```python
from build123d import *

# Parameters (mm, degrees)
F0_W      = 50
F0_H      = 81
F1_DEPTH  = 2
F0_H_2    = 3.6
F2_DEPTH  = 3.6
F4_R      = 1.75
F5_DEPTH  = 2
F3_R      = 1.75
F6_DEPTH  = 2
F1_FACE_W = 50
F1_FACE_H = 2
F7_DEPTH  = 6


with BuildPart() as f1:
    # F0 (on Front) → F1 (new body)
    with BuildSketch(Plane.XZ):
        with Locations((25, 40.5)):
            Rectangle(F0_W, F0_H)
    extrude(amount=F1_DEPTH)

    # F0 (on Front) → F2 (join)
    with BuildSketch(Plane.XZ):
        with Locations((25, 82.8)):
            Rectangle(F0_W, F0_H_2)
    extrude(amount=F2_DEPTH)

    # F4 (on face) → F5 (join)
    with BuildSketch(Plane(origin=(0, 0, 0), x_dir=(0, -1, 0), z_dir=(-1, 0, 0))):
        with Locations((1.783865, 82.8)):
            Circle(F4_R)
    extrude(amount=F5_DEPTH)

    # F3 (on face) → F6 (join)
    with BuildSketch(Plane.YZ.offset(50)):
        with Locations((-1.783865, 82.8)):
            Circle(F3_R)
    extrude(amount=F6_DEPTH)

    # F1_face (on face) → F7 (join)
    with BuildSketch(Plane(origin=(25, -1, 0), x_dir=(1, 0, 0), z_dir=(0, 0, -1))):
        Rectangle(F1_FACE_W, F1_FACE_H)
    extrude(amount=F7_DEPTH)


solid = f1.part
```
Check sheet for the modelled part. Datum: model origin and axes. Units: mm. A direction names the side the tool comes from. Coordinates: 2 decimals unless noted, no trailing zeros. Order: outer loops, then holes, each group sorted by start corner. A loop starts at its lowest first (then second) coordinate and runs counter-clockwise, first axis right, second up. Notation, with made-up numbers: (57, -1) -> (71, -1) arc R24 ccw to (71, 15) -> close; hole circle Ø8 at (-24.5, 43.5). An arc over 180 degrees is marked (long way). Write each question's results on one line, items separated by ' | '. Start each with the question number.
1) Depth check by flat-ended pin: pin 1 (1 mm diameter, centred on y = -1, z = 45.5, fed in from -X); pin 2 (1.5 mm diameter, centred on y = -3, z = 44.5, fed in from -X); pin 3 (4 mm diameter, centred on x = 17.5, z = 12.5, fed in from -Y). Enter the tip coordinate at first touch or a pass-through.
2) Section check A-A (x = 14). Enter the section's corners in (y, z), and give its area (3 significant figures).
3) Set-up check for faces 1 (the face through (25, -3, 81)), 2 (the face through (-0.986, -1.404, 81.092)), 3 (the face through (51, -2.2, 81.1)): record each of +Z, -Z, +X, -X, +Y, -Y from which the full face is reachable in a straight line by a thin tool's end or side.
4) Section check C-C (z = 75.5). Enter the section's corners in (x, y), and give its area (3 significant figures).
5) Material ranges on line 1 along Y through (x, z) = (32.5, 9); line 2 along Z through (x, y) = (5, -2.5); line 3 along X through (y, z) = (-1.05, 52.5), recorded low to high.
6) Section check B-B (y = -0.9). Enter the section's corners in (x, z).
Checked values:
1) pin 1: x = 0 | pin 2: through | pin 3: y = -2
2) outline: (-3.6, 81) -> (-2, 81) -> (-2, -6) -> (0, -6) -> (0, 84.6) -> (-3.6, 84.6) -> close | area: 187 mm²
3) face 1: -Z, +X, -X, -Y | face 2: -X | face 3: +X
4) outline: (0, -2) -> (50, -2) -> (50, 0) -> (0, 0) -> close | area: 100 mm²
5) line 1: -2 to 0 | line 2: 81 to 84.6 | line 3: 0 to 50
6) outline: (-2, 81.29) -> (0, 81.29) -> (0, -6) -> (50, -6) -> (50, 81.29) -> (52, 81.29) -> (52, 84.31) -> (50, 84.31) -> (50, 84.6) -> (0, 84.6) -> (0, 84.31) -> (-2, 84.31) -> close
